```python
from build123d import *

# Parameters (mm, degrees)
SKETCH1_W                  = 25.4
SKETCH1_H                  = 28.575
BOSS_EXTRUDE1_DEPTH        = 12.7
SKETCH3_W                  = 25.4
SKETCH3_H                  = 9.525
CUT_EXTRUDE1_DEPTH         = 9.525
SKETCH2_R                  = 3.175
CUT_EXTRUDE2_DEPTH         = 23.950221268
F_6_32_TAPPED_HOLE1_REACH  = 28.182
F_6_32_TAPPED_HOLE1_BORE_R = 1.35255
F_6_CLEARANCE_HOLE1_D      = 3.7973


with BuildPart() as part:
    # Sketch1 → Boss-Extrude1 (new body)
    with BuildSketch(Plane.XY):
        Rectangle(SKETCH1_W, SKETCH1_H)
    extrude(amount=BOSS_EXTRUDE1_DEPTH)

    # Sketch3 → Cut-Extrude1 (cut)
    with BuildSketch(Plane.XY.offset(12.7)):
        with Locations((0, -9.525)):
            Rectangle(SKETCH3_W, SKETCH3_H)
        with Locations((0, 9.525)):
            Rectangle(SKETCH3_W, SKETCH3_H)
    extrude(amount=-CUT_EXTRUDE1_DEPTH, mode=Mode.SUBTRACT)

    # Sketch2 → Cut-Extrude2 (cut, through all)
    with BuildSketch(Plane.XY.offset(12.7)):
        with Locations((-6.35, -0.3175)):
            Circle(SKETCH2_R)
    extrude(amount=-CUT_EXTRUDE2_DEPTH, mode=Mode.SUBTRACT)

    # #6-32 Tapped Hole1 bore → #6-32 Tapped Hole1 (cut, up to next)
    with BuildSketch(Plane(origin=(0, 4.7625, 0), x_dir=(1, 0, 0), z_dir=(0, 1, 0)), mode=Mode.PRIVATE) as f_6_32_tapped_hole1_sk1:
        with Locations((-6.35, -7.9375)):
            Circle(F_6_32_TAPPED_HOLE1_BORE_R)
    f_6_32_tapped_hole1_tool1 = extrude(f_6_32_tapped_hole1_sk1.sketch, amount=-F_6_32_TAPPED_HOLE1_REACH, mode=Mode.PRIVATE) & part.part
    add(f_6_32_tapped_hole1_tool1.solids().sort_by_distance((-6.35, 4.7625, 7.9375))[0], mode=Mode.SUBTRACT)

    # #6 Clearance Hole1 (through all)
    with Locations(Plane.XY.offset(3.175)):
        with Locations((-6.35, 9.525), (6.35, 9.525), (-6.35, -8.5725)):
            Hole(F_6_CLEARANCE_HOLE1_D / 2)


solid = part.part
```
Design review of the part built by this model. Coordinates are the model's own, in mm. A direction names the side the tool comes from. Give positions to 0.01 mm unless a question says otherwise; leave off trailing zeros. Order: outer loops, then holes, each group sorted by start corner. A loop starts at its lowest first (then second) coordinate and runs counter-clockwise, first axis right, second up. Notation, with made-up numbers: M 43,9.25 L 92,9.25 A10 cw 92,24.25 Z; hole C -37.5,-23.75 d10. An arc over 180 degrees is marked long. One line per question, with ' | ' between items. Start each with the question number.
Q1. We need section A-A (x = -6.35). Write out the cut boundary in (y, z) (1 decimal).
Q2. For pin 1 Ø3 at (x, y) = (1, 7) entering from +Z (3 decimals); pin 2 Ø1 at (x, z) = (6.5, 5.5) entering from +Y; pin 3 Ø3.5 at (x, y) = (-6.35, -8.57) entering from +Z; pin 4 Ø1.6 at (x, z) = (-6.35, 7.94) entering from -Y, all flat-tipped, find the tip position at first contact; note any pin that passes through.
Q3. We need section B-B (x = 6.35). Write out the cut boundary in (y, z) (1 decimal).
Q4. We need section C-C (z = 2). State how many separate pieces and enclosed holes the cut face has, plus the area to 3 significant figures.
Q5. Machinability: for faces 1 (the face through (-6.64, 3.67, 9.26)), 2 (the face through (-8.16, 10.1, 1.57)), 3 (the face through (0, 4.762, 8)), 4 (the face through (0, -4.762, 8)), 5 (the face through (0, -14.288, 2)), which of the approach directions +Z, -Z, +X, -X, +Y, -Y give a long, thin tool a straight path to every point of the face, cutting with its end or side? Answer none if there is none.
Q6. For L1, parallel to Y at x = -6.35, z = 0.9; L2, parallel to Y at x = 6.35, z = 2.15; L3, parallel to Y at x = -6.35, z = 10.25, list the stretches that pass through material, from the lowest coordinate up. Write a range as [from, to].
Q7. The part is to be moulded in two halves that separate along Y. For faces 6 (the face through (12.7, 0, 5)), 7 (the face through (-5.938, -10.426, 1.565)), 8 (the face through (0, 14.288, 2)), say which applies: +Y half, -Y half, draft (parallel to the pull), parting line (faces both ways), or undercut.
Q8. We need section D-D (x = -11). Write out the cut boundary in (y, z) (1 decimal), plus the area to 3 significant figures.
Returned:
1) outline: M -14.3,0 L -10.5,0 L -10.5,3.2 L -14.3,3.2 Z; M -6.7,0 L -3.5,0 L -3.5,12.7 L -4.8,12.7 L -4.8,3.2 L -6.7,3.2 Z; M 2.9,0 L 7.6,0 L 7.6,3.2 L 4.8,3.2 L 4.8,6.6 L 2.9,6.6 Z; M 2.9,9.3 L 4.8,9.3 L 4.8,12.7 L 2.9,12.7 Z; M 11.4,0 L 14.3,0 L 14.3,3.2 L 11.4,3.2 Z
2) pin 1: z = 3.175 | pin 2: y = 4.76 | pin 3: through | pin 4: y = -4.76
3) outline: M -14.3,0 L 7.6,0 L 7.6,3.2 L 4.8,3.2 L 4.8,12.7 L -4.8,12.7 L -4.8,3.2 L -14.3,3.2 Z; M 11.4,0 L 14.3,0 L 14.3,3.2 L 11.4,3.2 Z
4) separate pieces: 1 | enclosed holes: 4 | area: 660 mm2
5) face 1: +Y | face 2: +Z, -Z | face 3: +Z, +X, -X, +Y | face 4: +Z, +X, -X, -Y | face 5: +Z, -Z, +X, -X, -Y
6) L1: [-14.29, -10.47], [-6.67, -3.49], [2.86, 7.63], [11.42, 14.29] | L2: [-14.29, 7.63], [11.42, 14.29] | L3: [-4.76, -3.49], [2.86, 4.76]
7) face 6: draft | face 7: undercut | face 8: +Y half
8) outline: M -14.3,0 L 14.3,0 L 14.3,3.2 L 4.8,3.2 L 4.8,12.7 L -4.8,12.7 L -4.8,3.2 L -14.3,3.2 Z | area: 181 mm2
